Read the model definition and answer for the solid it produces. Units are mm, in the model's axes. Face numbers are marked on the shaded views. Coordinates: 2 decimals unless noted, no trailing zeros. Write each loop counter-clockwise with the first axis right and the second up, starting at its lowest first coordinate (ties: lowest second). Pieces come first, ordered by that corner, then holes. Notation, with made-up numbers: (34.25, 9) -> (46.25, 9) arc R22 cw to (46.25, 45) -> close; hole circle Ø5 at (0, -7). An arc over 180 degrees is marked (long way). Write item = value, one per line. Start each with the question number.
1) Section D-D (y = -4) is taken. Determine the outline of the cut face in (x, z).
2) Section B-B (x = 18) is taken. Determine the outline of the cut face in (y, z), plus the area to 3 significant figures.
3) Section C-C (x = -3) is taken. Determine the outline of the cut face in (y, z), plus the area to 3 significant figures.
4) Find the intervals of material crossed by line 1 along Y through (x, z) = (-4.5, 4.3); line 2 along Y through (x, z) = (18, 1.2); line 3 along X through (y, z) = (-18.5, 1.7), in increasing order. Write a range as from..to.
5) For a pull along X with two mould halves and no side action, classify the marked faces 1 and 2 as released by +X, released by -X, zero draft, split by the parting line, or undercut.
6) Section A-A (y = 47.5) is taken. Determine the outline of the cut face in (x, z), plus the area to 3 significant figures.
7) Flat-ended cylindrical pins translate along their axes: pin 1 Ø1 at (x, y) = (-5.5, -0.5) entering from -Z; pin 2 Ø1.5 at (x, y) = (0, -1) entering from +Z. Find the tip coordinate at first contact, or state that the pin passes through.
from build123d import *

# Parameters (mm, degrees)
SKETCH_1_W          = 45
SKETCH_1_H          = 100
EXTRUDE_1_DEPTH     = 5
SKETCH_2_W          = 41
SKETCH_2_H          = 60
CUT_EXTRUDE_1_DEPTH = 1
SKETCH_5_W          = 45
SKETCH_5_H          = 5
EXTRUDE_2_DEPTH     = 5
SKETCH_4_R          = 1.6
CUT_EXTRUDE_4_DEPTH = 10
SKETCH_3_R          = 1.6
CUT_EXTRUDE_7_DEPTH = 10


with BuildPart() as part:
    # 草图1 → 凸台-拉伸1 (new body)
    with BuildSketch(Plane.XY):
        Rectangle(SKETCH_1_W, SKETCH_1_H)
    extrude(amount=EXTRUDE_1_DEPTH)

    # 草图2 → 切除-拉伸1 (cut)
    with BuildSketch(Plane.XY.offset(5)):
        Rectangle(SKETCH_2_W, SKETCH_2_H)
    extrude(amount=-CUT_EXTRUDE_1_DEPTH, mode=Mode.SUBTRACT)

    # 草图5 → 凸台-拉伸2 (add)
    with BuildSketch(Plane.XY.offset(5)):
        with Locations((0, 52.5)):
            Rectangle(SKETCH_5_W, SKETCH_5_H)
        with Locations((0, -52.5)):
            Rectangle(SKETCH_5_W, SKETCH_5_H)
    extrude(amount=-EXTRUDE_2_DEPTH)

    # 草图4 → 切除-拉伸4 (cut)
    with BuildSketch(Plane.XY.offset(5)):
        with Locations((-17.5, 47.5)):
            Circle(SKETCH_4_R)
        with Locations((17.5, 47.5)):
            Circle(SKETCH_4_R)
        with Locations((-17.5, -47.5)):
            Circle(SKETCH_4_R)
        with Locations((17.5, -47.5)):
            Circle(SKETCH_4_R)
    extrude(amount=-CUT_EXTRUDE_4_DEPTH, mode=Mode.SUBTRACT)

    # 草图3 → 切除-拉伸7 (cut)
    with BuildSketch(Plane.XY.offset(4)):
        with BuildLine():
            ThreePointArc((-17.833531825, 16.4), (-16.702160975, 16.86862915), (-16.233531825, 18))
            Line((-16.233531825, 18), (-17.833531825, 18))
            Line((-17.833531825, 18), (-17.833531825, 16.4))
        make_face()
        with BuildLine():
            Line((-17.833531825, 18), (-16.233531825, 18))
            ThreePointArc((-16.233531825, 18), (-18.964902675, 19.13137085), (-17.833531825, 16.4))
            Line((-17.833531825, 16.4), (-17.833531825, 18))
        make_face()
        with Locations((-17.833531825, -18)):
            Circle(SKETCH_3_R)
        with Locations((18, -18)):
            Circle(SKETCH_3_R)
        with Locations((18.166468175, 18)):
            Circle(SKETCH_3_R)
    extrude(amount=-CUT_EXTRUDE_7_DEPTH, mode=Mode.SUBTRACT)


solid = part.part
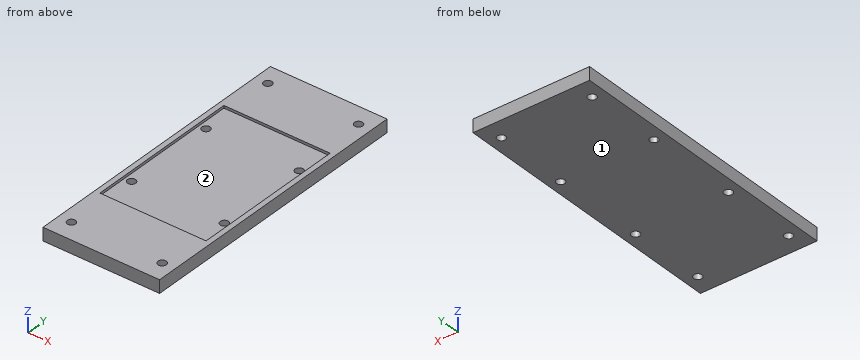
Answer key:
q1.outline = (-22.5, 0) -> (22.5, 0) -> (22.5, 5) -> (20.5, 5) -> (20.5, 4) -> (-20.5, 4) -> (-20.5, 5) -> (-22.5, 5) -> close
q2.outline = (-55, 0) -> (-49.02, 0) -> (-49.02, 5) -> (-55, 5) -> close; (-45.98, 0) -> (-19.6, 0) -> (-19.6, 4) -> (-30, 4) -> (-30, 5) -> (-45.98, 5) -> close; (-16.4, 0) -> (16.41, 0) -> (16.41, 4) -> (-16.4, 4) -> close; (19.59, 0) -> (45.98, 0) -> (45.98, 5) -> (30, 5) -> (30, 4) -> (19.59, 4) -> close; (49.02, 0) -> (55, 0) -> (55, 5) -> (49.02, 5) -> close
q2.area = 434 mm^2
q3.outline = (-55, 0) -> (55, 0) -> (55, 5) -> (30, 5) -> (30, 4) -> (-30, 4) -> (-30, 5) -> (-55, 5) -> close
q3.area = 490 mm^2
q4.line_1 = -55..-30, 30..55
q4.line_2 = -55..-49.02, -45.98..-19.6, -16.4..16.41, 19.59..45.98, 49.02..55
q4.line_3 = -22.5..-19.35, -16.31..16.48, 19.52..22.5
q5.face_1 = zero draft
q5.face_2 = undercut
q6.outline = (-22.5, 0) -> (-19.1, 0) -> (-19.1, 5) -> (-22.5, 5) -> close; (-15.9, 0) -> (15.9, 0) -> (15.9, 5) -> (-15.9, 5) -> close; (19.1, 0) -> (22.5, 0) -> (22.5, 5) -> (19.1, 5) -> close
q6.area = 193 mm^2
q7.pin_1 = 0
q7.pin_2 = 4
